from build123d import *

# Parameters (mm, degrees)
BOX022_W          = 30
BOX022_H          = 20
BOX022_DEPTH      = 9.2
BOX011_W          = 26
BOX011_H          = 12
BOX011_DEPTH      = 5.2
CYLINDER005_R     = 0.75
CYLINDER005_DEPTH = 7
ARRAY005_X_COUNT  = 8
ARRAY005_X_PITCH  = 2.6
ARRAY005_Y_COUNT  = 2
ARRAY005_Y_PITCH  = 1
BOX010_W          = 20.8
BOX010_H          = 18
BOX010_DEPTH      = 7.2


with BuildPart() as obj1:
    # Box022 → Box022 (new body)
    with BuildSketch(Plane(origin=(-1, -2, 3.6), x_dir=(1, 0, 0), z_dir=(0, 0, 1))):
        with Locations((15, 10)):
            Rectangle(BOX022_W, BOX022_H)
    extrude(amount=BOX022_DEPTH)


with BuildPart() as cube_10_base007:
    # Box011 → Box011 (new body)
    with BuildSketch(Plane(origin=(0, 6, 1), x_dir=(1, 0, 0), z_dir=(0, 0, 1))):
        with Locations((13, 6)):
            Rectangle(BOX011_W, BOX011_H)
    extrude(amount=BOX011_DEPTH)


with BuildPart() as array005:
    # Cylinder005 → Cylinder005 (new body)
    with BuildSketch(Plane(origin=(1.3, -1, 3.6), x_dir=(1, 0, 0), z_dir=(0, 1, 0))):
        Circle(CYLINDER005_R)
    extrude(amount=CYLINDER005_DEPTH)

    # Array005 X: Array005 ×8


with BuildPart() as array005_1:
    add(array005.part)
    with Locations(*[(i * ARRAY005_X_PITCH, 0, 0) for i in range(1, ARRAY005_X_COUNT)]):
        add(array005.part)

    # Array005 Y: Array005 ×2


with BuildPart() as array005_2:
    add(array005_1.part)
    with Locations(*[(0, i * ARRAY005_Y_PITCH, 0) for i in range(1, ARRAY005_Y_COUNT)]):
        add(array005_1.part)


with BuildPart() as obj2:
    # Box010 → Box010 (new body)
    with BuildSketch(Plane.XY):
        with Locations((10.4, 9)):
            Rectangle(BOX010_W, BOX010_H)
    extrude(amount=BOX010_DEPTH)

    # Cut011: cut Array005
    add(array005_2.part, mode=Mode.SUBTRACT)

    # Cut010: cut cube_10_base007
    add(cube_10_base007.part, mode=Mode.SUBTRACT)

    # Cut021: cut obj1
    add(obj1.part, mode=Mode.SUBTRACT)


solid = obj2.part
Design review of the part built by this model. Coordinates are the model's own, in mm. A direction names the side the tool comes from. Coordinates: 2 decimals unless noted, no trailing zeros. Write each loop counter-clockwise with the first axis right and the second up, starting at its lowest first coordinate (ties: lowest second). Pieces come first, ordered by that corner, then holes. Notation, with made-up numbers: (-17, -4.75) - (36, -4.75) arc R23 cw to (36, 5.25) - close; hole circle Ø5 at (14.5, 8.5). An arc over 180 degrees is marked (long way). Use one line per item in the form item = value.
Q1. Consider section A-A (y = 1.5). Write out the cut boundary in (x, z), plus the area to 3 significant figures.
Taken from the geometry:
outline = (0, 0) - (20.8, 0) - (20.8, 3.6) - (20.25, 3.6) arc R0.75 cw to (18.75, 3.6) - (17.65, 3.6) arc R0.75 cw to (16.15, 3.6) - (15.05, 3.6) arc R0.75 cw to (13.55, 3.6) - (12.45, 3.6) arc R0.75 cw to (10.95, 3.6) - (9.85, 3.6) arc R0.75 cw to (8.35, 3.6) - (7.25, 3.6) arc R0.75 cw to (5.75, 3.6) - (4.65, 3.6) arc R0.75 cw to (3.15, 3.6) - (2.05, 3.6) arc R0.75 cw to (0.55, 3.6) - (0, 3.6) - close
area = 67.8 mm^2
Q2. Consider section C-C (z = 3.3). Count the separate pieces of the cut face and the enclosed holes in it, plus the area to 3 significant figures.
Taken from the geometry:
separate_pieces = 9
enclosed_holes = 0
area = 58.8 mm^2
Q3. Machinability: for faces 1 (the flat face through (0, 6.9, 0.6)), 2 (the flat face through (10, 12, 1)), which of the approach directions +Z, -Z, +X, -X, +Y, -Y give a long, thin tool a straight path to every point of the face, cutting with its end or side? Answer none if there is none.
Taken from the geometry:
face_1 = +Z, -Z, -X, +Y, -Y
face_2 = +Z, +X, -X, +Y
Q4. Consider section B-B (x = 19.5). Write out the cut boundary in (y, z).
Taken from the geometry:
outline = (0, 0) - (18, 0) - (18, 1) - (6, 1) - (6, 2.85) - (0, 2.85) - close
Q5. Insertion check: pin 1 Ø5 at (x, y) = (6.5, 2) entering from -Z; pin 2 Ø1.3 at (x, z) = (12.5, 2.5) entering from +Y. Each pin has a flat end and moves straight along its axis. Give the tip position at first contact, or say it passes through.
Taken from the geometry:
pin_1 = 0
pin_2 = 6
Q6. For probe 1 along Z at (x, y) = (7.5, 13); probe 2 along Y at (x, z) = (11.25, 2.2); probe 3 along Z at (x, y) = (16.5, 4.5), list the stretches that pass through material, from the lowest coordinate up.
Taken from the geometry:
probe_1 = 0 to 1
probe_2 = 0 to 6
probe_3 = 0 to 2.97
Q7. Consider section D-D (x = 8). Write out the cut boundary in (y, z).
Taken from the geometry:
outline = (0, 0) - (18, 0) - (18, 1) - (6, 1) - (6, 3.6) - (0, 3.6) - close
Q8. The part is to be moulded in two halves that separate along X. For faces 3 (the flat face through (10.4, 3, 3.6)), 4 (the cylindrical face through (19.52, 2.96, 2.85)), 5 (the flat face through (20.8, 6.9, 0.6)), say which applies: +X half, -X half, draft (parallel to the pull), parting line (faces both ways), or undercut.
Taken from the geometry:
face_3 = draft
face_4 = undercut
face_5 = +X half
